Input: part model. Units: mm. Frame: model coordinates. A direction names the side the tool comes from. Give positions to 0.01 mm unless a question says otherwise; leave off trailing zeros. Write each loop counter-clockwise with the first axis right and the second up, starting at its lowest first coordinate (ties: lowest second). Pieces come first, ordered by that corner, then holes. Notation, with made-up numbers: (9.25, 68.25) - (38.25, 68.25) arc R30 ccw to (38.25, 94.25) - close; hole circle Ø7 at (2, -6.75). An arc over 180 degrees is marked (long way). Answer as CSV lines item,"result".
```python
from build123d import *

# Parameters (mm, degrees)
F0_W     = 66.548
F0_H     = 34.544
F1_DEPTH = 101.854
F2_T     = -1.778
F3_R     = 1.778
F4_R     = 14.8402874642
F5_DEPTH = 23.89732
F6_DEPTH = 25.4
F7_R     = 5.08


with BuildPart() as f1:
    # F0 (on Top) → F1 (new body)
    with BuildSketch(Plane.XY):
        with Locations((0, 6.62432)):
            Rectangle(F0_W, F0_H)
    extrude(amount=F1_DEPTH)

    # F2
    f2_openings = [f1.faces().sort_by_distance(p)[0] for p in [
        (0, 6.62432, 101.854),
    ]]
    offset(amount=F2_T, openings=f2_openings)

    # F3
    f3_edges = [f1.edges().sort_by_distance(p)[0] for p in [
        (-33.274, 23.89632, 50.927),
        (-33.274, -10.64768, 50.927),
        (33.274, -10.64768, 50.927),
        (33.274, 23.89632, 50.927),
    ]]
    fillet(f3_edges, radius=F3_R)

    # F4 (on Front) → F5 (cut, through all)
    with BuildSketch(Plane.XZ):
        with Locations((0, 102.1052822471)):
            Circle(F4_R)
    extrude(amount=-F5_DEPTH, mode=Mode.SUBTRACT)

    # F4 (on Front) → F6 (cut)
    with BuildSketch(Plane.XZ):
        with Locations((0, 102.1052822471)):
            Circle(F4_R)
    extrude(amount=F6_DEPTH, mode=Mode.SUBTRACT)

    # F7
    f7_edges = [f1.edges().sort_by_distance(p)[0] for p in [
        (-14.83816, 23.00732, 101.854),
        (14.83816, 23.00732, 101.854),
        (14.83816, -9.75868, 101.854),
        (-14.83816, -9.75868, 101.854),
    ]]
    fillet(f7_edges, radius=F7_R)


solid = f1.part
```
Item 1: Reachability of faces 5 (the face through (0, 7, 0)), 6 (the face through (31.496, 6, 51)), 7 (the face through (-16.16, -9.75, 100.85)) from +Z, -Z, +X, -X, +Y, -Y: full face, straight path, thin tool, end or side. Return the list, or none.
The answers:
face 5,"-Z, +X, -X, +Y, -Y"
face 6,"+Z"
face 7,"+Z, +Y, -Y"
Item 2: Mould query, pull axis X, two halves, no side actions, for faces 1 (the face through (0, -8.87, 51)), 2 (the face through (0, 23.896, 50)), 3 (the face through (33.274, 6, 50)), 4 (the face through (-16.16, 22.99, 100.85)). Classes: +X half, -X half, draft (parallel to the pull), parting line (faces both ways), or undercut.
The answers:
face 1,"undercut"
face 2,"draft"
face 3,"+X half"
face 4,"undercut"
Item 3: Contact query for a flat-ended pin moving along its axis: pin 1 (15.5 mm diameter, centred on x = 0.5, y = 7.5, fed in from +Z). Output: stop coordinate, or through.
The answers:
pin 1,"z = 1.78"
Item 4: Cut plane D-D on z = 77.5. Return the cut outline in (x, y), plus the area to 3 significant figures.
The answers:
outline,"(-33.27, -8.87) arc R1.78 ccw to (-31.5, -10.65) - (31.5, -10.65) arc R1.78 ccw to (33.27, -8.87) - (33.27, 22.12) arc R1.78 ccw to (31.5, 23.9) - (-31.5, 23.9) arc R1.78 ccw to (-33.27, 22.12) - close; hole (-31.5, -8.87) - (31.5, -8.87) - (31.5, 22.12) - (-31.5, 22.12) - close"
area,"344 mm²"
Item 5: Cut plane B-B on z = 95.5. Return the cut outline in (x, y).
The answers:
outline,"(-33.27, -8.87) arc R1.78 ccw to (-31.5, -10.65) - (-13.29, -10.65) - (-13.29, -8.87) - (-31.5, -8.87) - (-31.5, 22.12) - (-13.29, 22.12) - (-13.29, 23.9) - (-31.5, 23.9) arc R1.78 ccw to (-33.27, 22.12) - close; (13.29, -10.65) - (31.5, -10.65) arc R1.78 ccw to (33.27, -8.87) - (33.27, 22.12) arc R1.78 ccw to (31.5, 23.9) - (13.29, 23.9) - (13.29, 22.12) - (31.5, 22.12) - (31.5, -8.87) - (13.29, -8.87) - close"
Item 6: Cut plane C-C on y = 2. Return the cut outline in (x, z).
The answers:
outline,"(-33.27, 0) - (33.27, 0) - (33.27, 101.85) - (31.5, 101.85) - (31.5, 1.78) - (-31.5, 1.78) - (-31.5, 101.85) - (-33.27, 101.85) - close"
Item 7: Ray query, line 1 (Y direction, x = -26.5, z = 97.5); line 2 (X direction, y = 7.5, z = 7); line 3 (Z direction, x = -4.5, y = -6.5). Return the intervals inside material, ascending. Write a range as from..to.
The answers:
line 1,"-10.65..-8.87, 22.12..23.9"
line 2,"-33.27..-31.5, 31.5..33.27"
line 3,"0..1.78"
Item 8: Cut plane A-A on x = 24. Return the cut outline in (y, z), plus the area to 3 significant figures.
The answers:
outline,"(-10.65, 0) - (23.9, 0) - (23.9, 101.85) - (22.12, 101.85) - (22.12, 1.78) - (-8.87, 1.78) - (-8.87, 101.85) - (-10.65, 101.85) - close"
area,"417 mm²"
